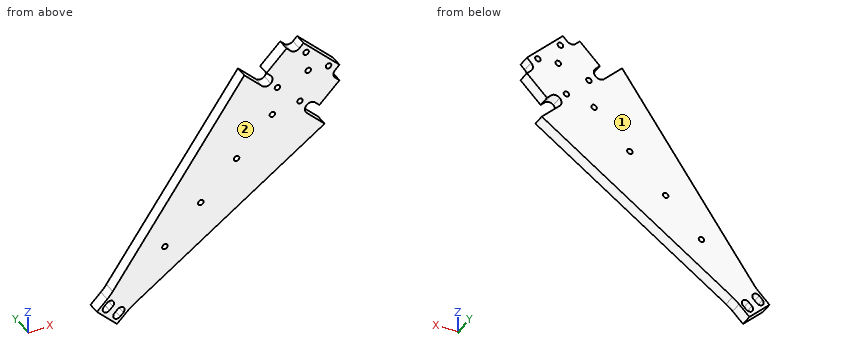
from build123d import *

# Parameters (mm, degrees)
BOSS_EXTRUDE1_DEPTH    = 3.175
FILLET1_R              = 25
M2_5_CLEARANCE_HOLE1_D = 2.9
FILLET2_R              = 3.175


with BuildPart() as part:
    # Sketch1 → Boss-Extrude1 (new, symmetric)
    with BuildSketch(Plane(origin=(0, 0, 0), x_dir=(1, 0, 0), z_dir=(0, 1, 0))):
        Polygon((12.993087104, -2.386485387), (2.386485387, -12.993087104), (9.457553198, -20.064154916), (80.256619665, -122.683026536), (91.985753398, -110.953892803), (96.475881458, -115.444020863), (91.985753398, -119.934148924), (102.592355115, -130.540750642), (107.082483176, -126.050622581), (111.572611236, -130.540750642), (130.540750642, -111.572611236), (126.050622581, -107.082483176), (130.540750642, -102.592355115), (119.934148924, -91.985753398), (115.444020863, -96.475881458), (110.953892803, -91.985753398), (122.683026536, -80.256619665), (20.064154916, -9.457553198), align=None)
        with BuildLine():
            Line((9.060159187, -11.622714162), (10.82792614, -13.390481115))
            ThreePointArc((10.82792614, -13.390481115), (10.82792614, -16.395684935), (7.82272232, -16.395684935))
            Line((7.82272232, -16.395684935), (6.054955367, -14.627917982))
            ThreePointArc((6.054955367, -14.627917982), (6.054955367, -11.622714162), (9.060159187, -11.622714162))
        make_face(mode=Mode.SUBTRACT)
        with BuildLine():
            Line((14.627917982, -6.054955367), (16.395684935, -7.82272232))
            ThreePointArc((16.395684935, -7.82272232), (16.395684935, -10.82792614), (13.390481115, -10.82792614))
            Line((13.390481115, -10.82792614), (11.622714162, -9.060159187))
            ThreePointArc((11.622714162, -9.060159187), (11.622714162, -6.054955367), (14.627917982, -6.054955367))
        make_face(mode=Mode.SUBTRACT)
    extrude(amount=BOSS_EXTRUDE1_DEPTH, both=True)

    # Fillet1
    fillet1_edges = [part.edges().sort_by_distance(p)[0] for p in [
        (9.457553198, 0, 20.064154916),
        (20.064154916, 0, 9.457553198),
    ]]
    fillet(fillet1_edges, radius=FILLET1_R)

    # M2.5 Clearance Hole1 (through all)
    with Locations(Plane(origin=(0, 3.175, 0), x_dir=(1, 0, 0), z_dir=(0, 1, 0))):
        with Locations((97.766351334, -109.663422927), (109.663422927, -97.766351334), (112.863081112, -124.760152706), (124.760152706, -112.863081112), (38.32518754, -38.32518754), (57.240293937, -57.240293937), (76.155400334, -76.155400334), (95.070506731, -95.070506731), (113.985613127, -113.985613127)):
            Hole(M2_5_CLEARANCE_HOLE1_D / 2)

    # Fillet2
    fillet2_edges = [part.edges().sort_by_distance(p)[0] for p in [
        (110.953892803, 0, 91.985753398),
        (115.444020863, 0, 96.475881458),
        (126.050622581, 0, 107.082483176),
        (107.082483176, 0, 126.050622581),
        (96.475881458, 0, 115.444020863),
        (91.985753398, 0, 110.953892803),
    ]]
    fillet(fillet2_edges, radius=FILLET2_R - 0.0001)  # a hair under: the kernel refuses the full size


solid = part.part
Geometry check sheet. Reference: the model listing, model coordinates, mm. Face numbers are marked on the shaded views. Give positions to 0.01 mm unless a question says otherwise; leave off trailing zeros. Order: outer loops, then holes, each group sorted by start corner. A loop starts at its lowest first (then second) coordinate and runs counter-clockwise, first axis right, second up.
1) Material ranges on probe 1 along Z at (x, y) = (124.5, -0.5); probe 2 along Z at (x, y) = (119.5, 1.75); probe 3 along X at (y, z) = (2, 117), recorded low to high.
Results are:
probe 1: z = 96.55 to 111.44, 114.29 to 117.61
probe 2: z = 78.06 to 83.44, 92.42 to 122.61
probe 3: x = 76.34 to 85.94, 94.75 to 125.11
2) Cross-section at B-B (y = -1.25). Give the number of separate pieces and of enclosed holes in the cut face, then the cut area to 3 significant figures.
Results are:
separate pieces: 1
enclosed holes: 11
area: 5,590 mm2
3) Gauge pin test, flat ends, axial feed: pin 1 (2 mm diameter, centred on y = 1, z = 108, fed in from -X); pin 2 (1.5 mm diameter, centred on x = 58.5, y = 2, fed in from -Z); pin 3 (2.5 mm diameter, centred on x = 97.77, z = 109.66, fed in from +Y); pin 4 (4.5 mm diameter, centred on x = 57.24, z = 57.24, fed in from +Y) (3 decimals). Record the tip position at first contact, or that the pin passes through.
Results are:
pin 1: stops at x = 69.44
pin 2: stops at z = 35.46
pin 3: passes through
pin 4: stops at y = 3.175
4) Cross-section at C-C (z = 64.5). Record the boundary of the cut face in (x, y) (3 decimals), then the cut area to 3 significant figures.
Results are:
outline: (40.115, -3.175) - (99.845, -3.175) - (99.845, 3.175) - (40.115, 3.175) - close
area: 379 mm2
5) Draft check along Y on the marked faces 1 and 2. Enter one of: released by +Y, released by -Y, zero draft, split by the parting line, or undercut.
Results are:
face 1: released by +Y
face 2: released by -Y
6) Cross-section at A-A (x = 68). Record the boundary of the cut face in (y, z) (3 decimals), then the cut area to 3 significant figures.
Results are:
outline: (-3.175, 42.53) - (3.175, 42.53) - (3.175, 104.918) - (-3.175, 104.918) - close
area: 396 mm2
